Verification items for the finished model (mm, model axes). A direction names the side the tool comes from. Round coordinates to 2 decimals unless told otherwise and drop trailing zeros. Order: outer loops, then holes, each group sorted by start corner. A loop starts at its lowest first (then second) coordinate and runs counter-clockwise, first axis right, second up. Notation, with made-up numbers: (14, -18) -> (21, -18) arc R8 ccw to (21, -13) -> close; hole circle Ø4 at (22, 18). An arc over 180 degrees is marked (long way). Put each result on its own line as item: value.
```python
from build123d import *

# Parameters (mm, degrees)
SKETCH_2_R = 5


with BuildPart() as part:
    # 草图1 → 旋转1 (revolve)
    with BuildSketch(Plane.XY):
        Polygon((0, 0), (-335, 0), (-335, 27), (-332, 30), (-20, 30), (-20, 50), (0, 50), align=None)
    revolve(axis=Axis((0, 0, 0), (-1, 0, 0)))

    # 草图2 → 旋转2 (revolve)
    with BuildSketch(Plane(origin=(0, 0, 0), x_dir=(1, 0, 0), z_dir=(0, 1, 0)), mode=Mode.PRIVATE) as revolve_2_sk:
        with Locations((4.5, 0)):
            Circle(SKETCH_2_R)
    revolve(revolve_2_sk.sketch.rotate(Axis((49.5, 0, 1000), (0, 0, -1)), 265.94519807), axis=Axis((49.5, 0, 1000), (0, 0, -1)))


solid = part.part
```
Item 1: Sectioned sample at C-C, the plane x = -172.5. Record the boundary of the cut face in (y, z), then the cut area to 3 significant figures.
Geometry check:
outline: circle Ø60 at (0, 0)
area: 2,830 mm2
Item 2: Sectioned sample at A-A, the plane y = 21.5. Give the number of separate pieces and of enclosed holes in the cut face, then the cut area to 3 significant figures.
Geometry check:
separate pieces: 3
enclosed holes: 0
area: 15,200 mm2
Item 3: Material ranges on line 1 along X through (y, z) = (-44, 20); line 2 along X through (y, z) = (23, 10.5); line 3 along Z through (x, y) = (-111, -1.5), recorded low to high.
Geometry check:
line 1: -20 to 0
line 2: -335 to 0
line 3: -29.96 to 29.96
Item 4: Sectioned sample at B-B, the plane z = -35. Record the boundary of the cut face in (x, y).
Geometry check:
outline: (-20, -35.71) -> (0, -35.71) -> (0, 35.71) -> (-20, 35.71) -> close
Item 5: Tool access check on faces 1 (the face through (-335, 0, 0)), 2 (the face through (-173.82, -29.97, -1.32)). Record the directions out of +Z, -Z, +X, -X, +Y, -Y that give a thin tool (end or side, any length) a straight path to the whole face; none if there is none.
Geometry check:
face 1: +Z, -Z, -X, +Y, -Y
face 2: -X
Item 6: Depth check by flat-ended pin: pin 1 Ø1 at (y, z) = (33.5, -30) entering from +X; pin 2 Ø1 at (y, z) = (-36.5, -6) entering from -X; pin 3 Ø3 at (x, z) = (-45, 25.5) entering from -Y. Enter the tip coordinate at first touch or a pass-through.
Geometry check:
pin 1: x = 0
pin 2: x = -20
pin 3: y = -18
